from build123d import *

# Parameters (mm, degrees)
SKETCH1_R           = 2
SKETCH1_W           = 18
SKETCH1_H           = 15
SKETCH1_R_2         = 0.5
SKETCH1_R_3         = 0.5706303
SKETCH1_W_2         = 15
BOSS_EXTRUDE1_DEPTH = 2
SKETCH1_3_W         = 5
SKETCH1_3_H         = 7
SKETCH1_3_H_2       = 5
BOSS_EXTRUDE2_DEPTH = 5
SKETCH1_4_W         = 18
SKETCH1_4_H         = 15
SKETCH1_4_W_2       = 15
BOSS_EXTRUDE3_DEPTH = 3


with BuildPart() as part:
    # Sketch1 → Boss-Extrude1 (new body)
    with BuildSketch(Plane.XY):
        Polygon((3.5, 7.35633001), (-62.5, 7.35633001), (-62.5, -1.64366999), (-57.5, -1.64366999), (-57.5, -8.64366999), (-62.5, -8.64366999), (-62.5, -23.12366999), (3.5, -23.12366999), (3.5, -13.64366999), (-1.5, -13.64366999), (-1.5, -8.64366999), (3.5, -8.64366999), (3.5, -6.64366999), (-1.5, -6.64366999), (-1.5, -1.64366999), (3.5, -1.64366999), align=None)
        with Locations((-59, -19.62366999)):
            Circle(SKETCH1_R, mode=Mode.SUBTRACT)
        with Locations((-46.157324482, -9.14366999)):
            Rectangle(SKETCH1_W, SKETCH1_H, mode=Mode.SUBTRACT)
        with Locations((0, -19.62366999)):
            Circle(SKETCH1_R, mode=Mode.SUBTRACT)
        with Locations((-56, 3.35633001)):
            Circle(SKETCH1_R_2, mode=Mode.SUBTRACT)
        with Locations((-54.5, 3.35633001)):
            Circle(SKETCH1_R_3, mode=Mode.SUBTRACT)
        with Locations((-53, 3.35633001)):
            Circle(SKETCH1_R_2, mode=Mode.SUBTRACT)
        with Locations((-51.5, 3.35633001)):
            Circle(SKETCH1_R_2, mode=Mode.SUBTRACT)
        with Locations((-50, 3.35633001)):
            Circle(SKETCH1_R_3, mode=Mode.SUBTRACT)
        with Locations((-48.5, 3.35633001)):
            Circle(SKETCH1_R_2, mode=Mode.SUBTRACT)
        with Locations((-47, 3.35633001)):
            Circle(SKETCH1_R_2, mode=Mode.SUBTRACT)
        with Locations((-59, 3.85633001)):
            Circle(SKETCH1_R, mode=Mode.SUBTRACT)
        with Locations((-56, 5.35633001)):
            Circle(SKETCH1_R_2, mode=Mode.SUBTRACT)
        with Locations((-54.5, 5.35633001)):
            Circle(SKETCH1_R_3, mode=Mode.SUBTRACT)
        with Locations((-53, 5.35633001)):
            Circle(SKETCH1_R_2, mode=Mode.SUBTRACT)
        with Locations((-51.5, 5.35633001)):
            Circle(SKETCH1_R_2, mode=Mode.SUBTRACT)
        with Locations((-50, 5.35633001)):
            Circle(SKETCH1_R_3, mode=Mode.SUBTRACT)
        with Locations((-48.5, 5.35633001)):
            Circle(SKETCH1_R_2, mode=Mode.SUBTRACT)
        with Locations((-47, 5.35633001)):
            Circle(SKETCH1_R_2, mode=Mode.SUBTRACT)
        with Locations((-45.5, 3.35633001)):
            Circle(SKETCH1_R_3, mode=Mode.SUBTRACT)
        with Locations((-44, 3.35633001)):
            Circle(SKETCH1_R_2, mode=Mode.SUBTRACT)
        with Locations((-42.5, 3.35633001)):
            Circle(SKETCH1_R_2, mode=Mode.SUBTRACT)
        with Locations((-41, 3.35633001)):
            Circle(SKETCH1_R_3, mode=Mode.SUBTRACT)
        with Locations((-39.5, 3.35633001)):
            Circle(SKETCH1_R_2, mode=Mode.SUBTRACT)
        with Locations((-38, 3.35633001)):
            Circle(SKETCH1_R_2, mode=Mode.SUBTRACT)
        with Locations((-36.5, 3.35633001)):
            Circle(SKETCH1_R_3, mode=Mode.SUBTRACT)
        with Locations((-35, 3.35633001)):
            Circle(SKETCH1_R_2, mode=Mode.SUBTRACT)
        with Locations((-33.5, 3.35633001)):
            Circle(SKETCH1_R_2, mode=Mode.SUBTRACT)
        with Locations((-32, 3.35633001)):
            Circle(SKETCH1_R_3, mode=Mode.SUBTRACT)
        with Locations((-30.5, 3.35633001)):
            Circle(SKETCH1_R_2, mode=Mode.SUBTRACT)
        with Locations((-45.5, 5.35633001)):
            Circle(SKETCH1_R_3, mode=Mode.SUBTRACT)
        with Locations((-44, 5.35633001)):
            Circle(SKETCH1_R_2, mode=Mode.SUBTRACT)
        with Locations((-42.5, 5.35633001)):
            Circle(SKETCH1_R_2, mode=Mode.SUBTRACT)
        with Locations((-41, 5.35633001)):
            Circle(SKETCH1_R_3, mode=Mode.SUBTRACT)
        with Locations((-39.5, 5.35633001)):
            Circle(SKETCH1_R_2, mode=Mode.SUBTRACT)
        with Locations((-38, 5.35633001)):
            Circle(SKETCH1_R_2, mode=Mode.SUBTRACT)
        with Locations((-36.5, 5.35633001)):
            Circle(SKETCH1_R_3, mode=Mode.SUBTRACT)
        with Locations((-35, 5.35633001)):
            Circle(SKETCH1_R_2, mode=Mode.SUBTRACT)
        with Locations((-33.5, 5.35633001)):
            Circle(SKETCH1_R_2, mode=Mode.SUBTRACT)
        with Locations((-32, 5.35633001)):
            Circle(SKETCH1_R_3, mode=Mode.SUBTRACT)
        with Locations((-30.5, 5.35633001)):
            Circle(SKETCH1_R_2, mode=Mode.SUBTRACT)
        with Locations((-17.247739958, -7.5)):
            Rectangle(SKETCH1_W_2, SKETCH1_H, mode=Mode.SUBTRACT)
        with Locations((-29, 3.35633001)):
            Circle(SKETCH1_R_2, mode=Mode.SUBTRACT)
        with Locations((-27.5, 3.35633001)):
            Circle(SKETCH1_R_3, mode=Mode.SUBTRACT)
        with Locations((-26, 3.35633001)):
            Circle(SKETCH1_R_2, mode=Mode.SUBTRACT)
        with Locations((-24.5, 3.35633001)):
            Circle(SKETCH1_R_2, mode=Mode.SUBTRACT)
        with Locations((-23, 3.35633001)):
            Circle(SKETCH1_R_3, mode=Mode.SUBTRACT)
        with Locations((-21.5, 3.35633001)):
            Circle(SKETCH1_R_2, mode=Mode.SUBTRACT)
        with Locations((-20, 3.35633001)):
            Circle(SKETCH1_R_2, mode=Mode.SUBTRACT)
        with Locations((-18.5, 3.35633001)):
            Circle(SKETCH1_R_3, mode=Mode.SUBTRACT)
        with Locations((-17, 3.35633001)):
            Circle(SKETCH1_R_2, mode=Mode.SUBTRACT)
        with Locations((-15.5, 3.35633001)):
            Circle(SKETCH1_R_2, mode=Mode.SUBTRACT)
        with Locations((-14, 3.35633001)):
            Circle(SKETCH1_R_3, mode=Mode.SUBTRACT)
        with Locations((-29, 5.35633001)):
            Circle(SKETCH1_R_2, mode=Mode.SUBTRACT)
        with Locations((-27.5, 5.35633001)):
            Circle(SKETCH1_R_3, mode=Mode.SUBTRACT)
        with Locations((-26, 5.35633001)):
            Circle(SKETCH1_R_2, mode=Mode.SUBTRACT)
        with Locations((-24.5, 5.35633001)):
            Circle(SKETCH1_R_2, mode=Mode.SUBTRACT)
        with Locations((-23, 5.35633001)):
            Circle(SKETCH1_R_3, mode=Mode.SUBTRACT)
        with Locations((-21.5, 5.35633001)):
            Circle(SKETCH1_R_2, mode=Mode.SUBTRACT)
        with Locations((-20, 5.35633001)):
            Circle(SKETCH1_R_2, mode=Mode.SUBTRACT)
        with Locations((-18.5, 5.35633001)):
            Circle(SKETCH1_R_3, mode=Mode.SUBTRACT)
        with Locations((-17, 5.35633001)):
            Circle(SKETCH1_R_2, mode=Mode.SUBTRACT)
        with Locations((-15.5, 5.35633001)):
            Circle(SKETCH1_R_2, mode=Mode.SUBTRACT)
        with Locations((-14, 5.35633001)):
            Circle(SKETCH1_R_3, mode=Mode.SUBTRACT)
        with Locations((-12.5, 3.35633001)):
            Circle(SKETCH1_R_2, mode=Mode.SUBTRACT)
        with Locations((-11, 3.35633001)):
            Circle(SKETCH1_R_2, mode=Mode.SUBTRACT)
        with Locations((-9.5, 3.35633001)):
            Circle(SKETCH1_R_3, mode=Mode.SUBTRACT)
        with Locations((-8, 3.35633001)):
            Circle(SKETCH1_R_2, mode=Mode.SUBTRACT)
        with Locations((-6.5, 3.35633001)):
            Circle(SKETCH1_R_2, mode=Mode.SUBTRACT)
        with Locations((-5, 3.35633001)):
            Circle(SKETCH1_R_3, mode=Mode.SUBTRACT)
        with Locations((-3.5, 3.35633001)):
            Circle(SKETCH1_R_2, mode=Mode.SUBTRACT)
        with Locations((-12.5, 5.35633001)):
            Circle(SKETCH1_R_2, mode=Mode.SUBTRACT)
        with Locations((-11, 5.35633001)):
            Circle(SKETCH1_R_2, mode=Mode.SUBTRACT)
        with Locations((-9.5, 5.35633001)):
            Circle(SKETCH1_R_3, mode=Mode.SUBTRACT)
        with Locations((-8, 5.35633001)):
            Circle(SKETCH1_R_2, mode=Mode.SUBTRACT)
        with Locations((-6.5, 5.35633001)):
            Circle(SKETCH1_R_2, mode=Mode.SUBTRACT)
        with Locations((-5, 5.35633001)):
            Circle(SKETCH1_R_3, mode=Mode.SUBTRACT)
        with Locations((-3.5, 5.35633001)):
            Circle(SKETCH1_R_2, mode=Mode.SUBTRACT)
        with Locations((0, 3.85633001)):
            Circle(SKETCH1_R, mode=Mode.SUBTRACT)
    extrude(amount=BOSS_EXTRUDE1_DEPTH)

    # Sketch1_3 → Boss-Extrude2 (add)
    with BuildSketch(Plane.XY):
        with Locations((-60, -5.14366999)):
            Rectangle(SKETCH1_3_W, SKETCH1_3_H)
        with Locations((1, -4.14366999)):
            Rectangle(SKETCH1_3_W, SKETCH1_3_H_2)
        with Locations((1, -11.14366999)):
            Rectangle(SKETCH1_3_W, SKETCH1_3_H_2)
    extrude(amount=BOSS_EXTRUDE2_DEPTH)

    # Sketch1_4 → Boss-Extrude3 (add)
    with BuildSketch(Plane.XY):
        with Locations((-46.157324482, -9.14366999)):
            Rectangle(SKETCH1_4_W, SKETCH1_4_H)
        with Locations((-17.247739958, -7.5)):
            Rectangle(SKETCH1_4_W_2, SKETCH1_4_H)
    extrude(amount=BOSS_EXTRUDE3_DEPTH)


solid = part.part
For this review, take the finished solid that the model builds, in its own axes (mm). A direction names the side the tool comes from. Coordinates: 2 decimals unless noted, no trailing zeros. Write each loop counter-clockwise with the first axis right and the second up, starting at its lowest first coordinate (ties: lowest second). Pieces come first, ordered by that corner, then holes. Notation, with made-up numbers: (-30.75, 44) -> (-7.75, 44) arc R21 cw to (-7.75, 49) -> close; hole circle Ø10 at (-3.5, -29). An arc over 180 degrees is marked (long way). Write each question's results on one line, items separated by ' | '. Start each with the question number.
1) For faces 4 (the face through (-57.5, -5, 3)), 5 (the face through (-57.153, -20.39, 0.986)), 6 (the face through (1, -8.644, 3)), list the 3-axis set-ups (+Z, -Z, +X, -X, +Y, -Y) from which the entire face can be reached by the end or side of a thin tool; tool diameter is ignored.
2) Insertion check: pin 1 (4 mm diameter, centred on x = -55, y = -5.5, fed in from +Z); pin 2 (1.8 mm diameter, centred on x = -36.5, y = 3.36, fed in from +Z); pin 3 (0.9 mm diameter, centred on y = -12, z = 3, fed in from -X); pin 4 (2.5 mm diameter, centred on x = -59, y = 3.86, fed in from -Z). Each pin has a flat end and moves straight along its axis. Give the tip position at first contact, or say it passes through.
3) The part is to be moulded in two halves that separate along X. For faces 1 (the face through (-31.456, 5.528, 0.986)), 2 (the face through (-62.5, -8, 1)), 3 (the face through (-60, -5, 5)), say which applies: +X half, -X half, draft (parallel to the pull), parting line (faces both ways), or undercut.
4) Wall thickness on L1, parallel to Y at x = -5, z = 1.3; L2, parallel to Y at x = -3.5, z = 0.3; L3, parallel to Z at x = -28.5, y = -8.5: over which ranges is each line inside the solid? List them lowest first. Write a range as [from, to].
5) Consider section C-C (y = -1). Write out the cut boundary in (x, z), plus the area to 3 significant figures.
6) Consider section B-B (y = -11.5). Write out the cut boundary in (x, z), plus the area to 3 significant figures.
7) Consider section A-A (z = 3.85). Write out the cut boundary in (x, y).
Geometry says:
1) face 4: +Z, +Y, -Y | face 5: +Z, -Z | face 6: +Z, +X
2) pin 1: z = 3 | pin 2: z = 2 | pin 3: x = -55.16 | pin 4: through
3) face 1: undercut | face 2: -X half | face 3: draft
4) L1: [-23.12, 2.79], [3.93, 4.79], [5.93, 7.36] | L2: [-23.12, 2.86], [3.86, 4.86], [5.86, 7.36] | L3: [0, 2]
5) outline: (-62.5, 0) -> (3.5, 0) -> (3.5, 2) -> (-9.75, 2) -> (-9.75, 3) -> (-24.75, 3) -> (-24.75, 2) -> (-62.5, 2) -> close | area: 147 mm^2
6) outline: (-62.5, 0) -> (3.5, 0) -> (3.5, 5) -> (-1.5, 5) -> (-1.5, 2) -> (-9.75, 2) -> (-9.75, 3) -> (-24.75, 3) -> (-24.75, 2) -> (-37.16, 2) -> (-37.16, 3) -> (-55.16, 3) -> (-55.16, 2) -> (-62.5, 2) -> close | area: 180 mm^2
7) outline: (-62.5, -8.64) -> (-57.5, -8.64) -> (-57.5, -1.64) -> (-62.5, -1.64) -> close; (-1.5, -13.64) -> (3.5, -13.64) -> (3.5, -8.64) -> (-1.5, -8.64) -> close; (-1.5, -6.64) -> (3.5, -6.64) -> (3.5, -1.64) -> (-1.5, -1.64) -> close
